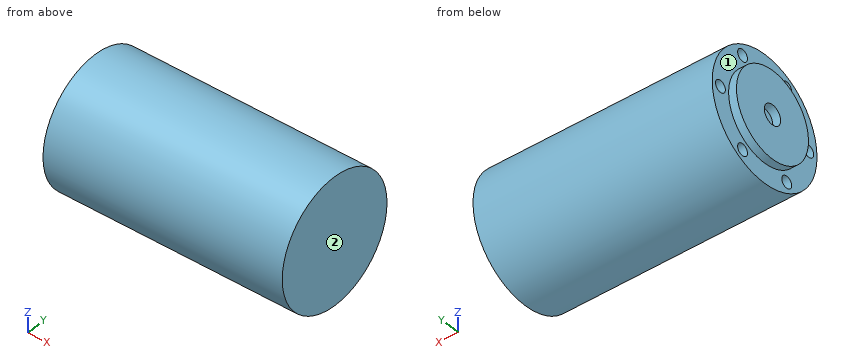
from build123d import *

# Parameters (mm, degrees)
SKETCH1_R           = 16
BOSS_EXTRUDE1_DEPTH = 61
SKETCH2_R           = 11
BOSS_EXTRUDE2_DEPTH = 2
SKETCH3_R           = 1.5
CUT_EXTRUDE1_DEPTH  = 4
SKETCH4_R           = 2.5
CUT_EXTRUDE2_DEPTH  = 2


with BuildPart() as part:
    # Sketch1 → Boss-Extrude1 (new body)
    with BuildSketch(Plane(origin=(0, 0, 0), x_dir=(0, 0, -1), z_dir=(1, 0, 0))):
        with Locations(Location((0, 0, 0), (0, 0, 180))):
            Circle(SKETCH1_R)
    extrude(amount=BOSS_EXTRUDE1_DEPTH)

    # Sketch2 → Boss-Extrude2 (add)
    with BuildSketch(Plane.ZY):
        Circle(SKETCH2_R)
    extrude(amount=BOSS_EXTRUDE2_DEPTH)

    # Sketch3 → Cut-Extrude1 (cut)
    with BuildSketch(Plane.ZY):
        with Locations((0, 13.5)):
            Circle(SKETCH3_R)
        with Locations((11.691342951, 6.75)):
            Circle(SKETCH3_R)
        with Locations((11.691342951, -6.75)):
            Circle(SKETCH3_R)
        with Locations((0, -13.5)):
            Circle(SKETCH3_R)
        with Locations((-11.691342951, -6.75)):
            Circle(SKETCH3_R)
        with Locations((-11.691342951, 6.75)):
            Circle(SKETCH3_R)
    extrude(amount=-CUT_EXTRUDE1_DEPTH, mode=Mode.SUBTRACT)

    # Sketch4 → Cut-Extrude2 (cut)
    with BuildSketch(Plane.ZY.offset(2)):
        Circle(SKETCH4_R)
    extrude(amount=-CUT_EXTRUDE2_DEPTH, mode=Mode.SUBTRACT)


solid = part.part
Geometry check sheet. Reference: the model listing, model coordinates, mm. Face numbers are marked on the shaded views. A direction names the side the tool comes from. Give positions to 0.01 mm unless a question says otherwise; leave off trailing zeros. Order: outer loops, then holes, each group sorted by start corner. A loop starts at its lowest first (then second) coordinate and runs counter-clockwise, first axis right, second up.
1) Gauge pin test, flat ends, axial feed: pin 1 (6 mm diameter, centred on x = 35.5, y = -12.5, fed in from +Z); pin 2 (5 mm diameter, centred on x = 42, y = 8, fed in from -Z) (3 decimals); pin 3 (5 mm diameter, centred on y = -10.5, z = 10, fed in from -X); pin 4 (5.5 mm diameter, centred on y = 0.5, z = -1, fed in from -X). Record the tip position at first contact, or that the pin passes through.
Results are:
pin 1: stops at z = 12.87
pin 2: stops at z = -15.025
pin 3: stops at x = 0
pin 4: stops at x = -2
2) Cross-section at D-D (z = -8.5). Record the boundary of the cut face in (x, y), then the cut area to 3 significant figures.
Results are:
outline: (-2, -6.98) - (0, -6.98) - (0, -13.56) - (61, -13.56) - (61, 13.56) - (0, 13.56) - (0, 6.98) - (-2, 6.98) - close
area: 1,680 mm2
3) Cross-section at C-C (x = 31). Record the boundary of the cut face in (y, z), then the cut area to 3 significant figures.
Results are:
outline: circle Ø32 at (0, 0)
area: 804 mm2
4) Material ranges on probe 1 along Y at (x, z) = (2.4, 0); probe 2 along X at (y, z) = (-6.5, -9); probe 3 along X at (y, z) = (7, 11), recorded low to high.
Results are:
probe 1: y = -16 to -15, -12 to 12, 15 to 16
probe 2: x = 0 to 61
probe 3: x = 4 to 61
5) Tool access check on the marked faces 1 and 2. Record the directions out of +Z, -Z, +X, -X, +Y, -Y that give a thin tool (end or side, any length) a straight path to the whole face; none if there is none.
Results are:
face 1: -X
face 2: +Z, -Z, +X, +Y, -Y
6) Cross-section at B-B (y = -13.5). Record the boundary of the cut face in (x, z), then the cut area to 3 significant figures.
Results are:
outline: (0, -8.59) - (61, -8.59) - (61, 8.59) - (0, 8.59) - (0, 1.5) - (4, 1.5) - (4, -1.5) - (0, -1.5) - close
area: 1,040 mm2
7) Cross-section at A-A (z = 0). Record the boundary of the cut face in (x, y), then the cut area to 3 significant figures.
Results are:
outline: (-2, -11) - (0, -11) - (0, -12) - (4, -12) - (4, -15) - (0, -15) - (0, -16) - (61, -16) - (61, 16) - (0, 16) - (0, 15) - (4, 15) - (4, 12) - (0, 12) - (0, 11) - (-2, 11) - (-2, 2.5) - (0, 2.5) - (0, -2.5) - (-2, -2.5) - close
area: 1,960 mm2
